Part print with two shaded views. Sizes in mm from the minimum x, y, z corner. A direction names the side the tool comes from. Round coordinates to 2 decimals unless told otherwise and drop trailing zeros. Order: outer loops, then holes, each group sorted by start corner. A loop starts at its lowest first (then second) coordinate and runs counter-clockwise, first axis right, second up. Notation, with made-up numbers: (75.5, 4) -> (93.5, 4) arc R17 ccw to (93.5, 27) -> close; hole circle Ø7 at (-36, 40). An arc over 180 degrees is marked (long way). Answer as a JSON object with one key per item and string values.
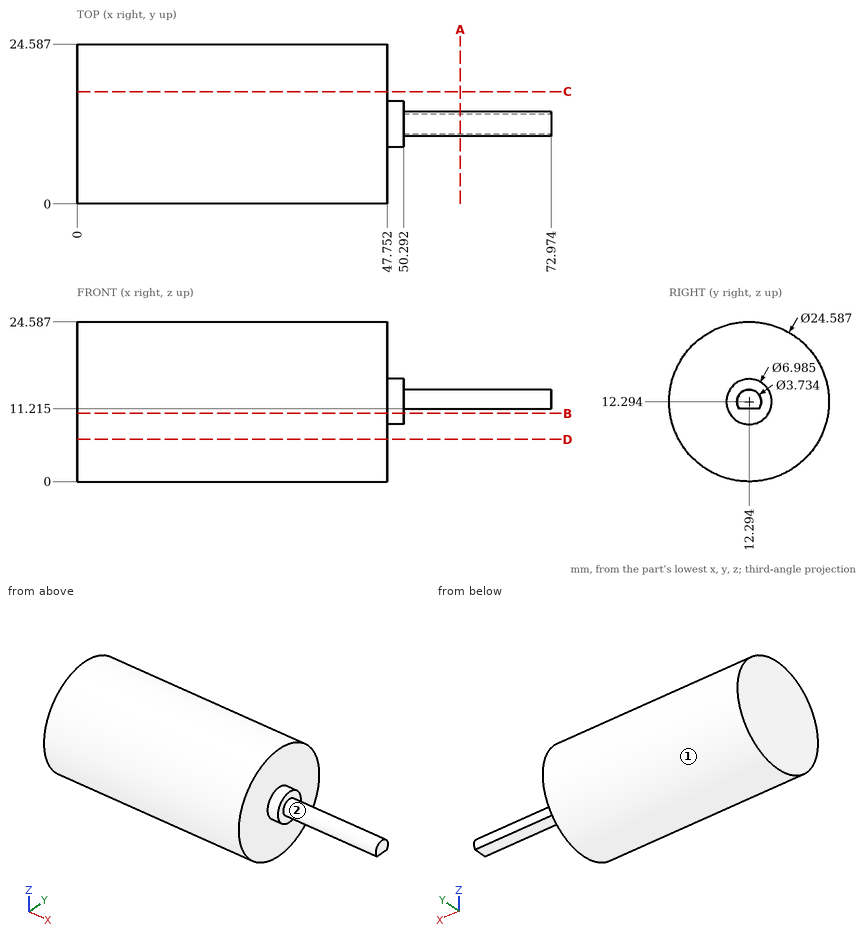
1) Cut at C-C, the plane y = 17.25. Give the cut face in (x, z), plus the area to 3 significant figures.
Checked values:
{"outline": "(0, 1.04) -> (47.75, 1.04) -> (47.75, 23.54) -> (0, 23.54) -> close", "area": "1,070 mm²"}
2) Cut at A-A, the plane x = 59. Give the cut face in (y, z) (1 decimal).
Checked values:
{"outline": "(10.8, 11.2) -> (13.8, 11.2) arc R1.9 ccw (long way) to start"}
3) Cut at B-B, the plane z = 10.5. Give the cut face in (x, y) (1 decimal), plus the area to 3 significant figures.
Checked values:
{"outline": "(0, 0.1) -> (47.8, 0.1) -> (47.8, 9.3) -> (50.3, 9.3) -> (50.3, 15.3) -> (47.8, 15.3) -> (47.8, 24.5) -> (0, 24.5) -> close", "area": "1,180 mm²"}
4) Cut at D-D, the plane z = 6.5. Give the cut face in (x, y), plus the area to 3 significant figures.
Checked values:
{"outline": "(0, 1.45) -> (47.75, 1.45) -> (47.75, 23.14) -> (0, 23.14) -> close", "area": "1,040 mm²"}
5) Which spindle directions (+Z, -Z, +X, -X, +Y, -Y) get a long thin tool onto all of the face, cutting with end or side? Do the marked faces 1 and 2. Say none if no direction does.
Checked values:
{"face 1": "+X, -X", "face 2": "+X"}
6) Flat gauge pins, fed straight in: pin 1 Ø2 at (x, y) = (31, 19) entering from +Z; pin 2 Ø6 at (x, y) = (61, 14.5) entering from -Z (1 decimal); pin 3 Ø5 at (x, y) = (18, 17) entering from +Z. Where does each tip first touch, or does it go through?
Checked values:
{"pin 1": "stops at z = 23.18", "pin 2": "stops at z = 11.2", "pin 3": "stops at z = 24.39"}
7) Probe L1, parallel to Z at x = 32, y = 12.75; L2, parallel to X at y = 1.5, z = 8.75; L3, parallel to Y at x = 26, z = 12. List the from-to ranges inside material, lowest first. Write a range as from..to.
Checked values:
{"L1": "z = 0.01..24.58", "L2": "x = 0..47.75", "L3": "y = 0..24.58"}
